Read the model definition and answer for the solid it produces. Units are mm, in the model's axes. Face numbers are marked on the shaded views. A direction names the side the tool comes from. Coordinates: 2 decimals unless noted, no trailing zeros. Order: outer loops, then holes, each group sorted by start corner. A loop starts at its lowest first (then second) coordinate and runs counter-clockwise, first axis right, second up. Notation, with made-up numbers: M -35.5,67.25 L -23.5,67.25 A20 cw -23.5,83.25 Z; hole C 89,-16.75 d9. An arc over 180 degrees is marked long. One line per question, with ' | ' between items. Start each with the question number.
1) A tool of negligible diameter and unlimited length cuts with its end or side. For the marked faces 1, 2 and 3, from which of +Z, -Z, +X, -X, +Y, -Y can it reach the whole face along a straight path? Write none if from no direction.
2) Find section D-D, the plane y = 0. Write down the section's boundary in (x, z), plus the area to 3 significant figures.
3) The mould has two halves that part along X. Classify the marked faces 4, 5 and 6: +X half, -X half, draft (parallel to the pull), parting line (faces both ways), or undercut.
4) Find section C-C, the plane x = 5. Write down the section's boundary in (y, z).
5) Given P1, Ø2, axis at x = 22, z = -2, coming from the -Y side; P2, Ø3, axis at x = 6, y = -0.5, coming from the -Z side; P3, Ø2, axis at y = 2, z = 5.5, coming from the -X side, each flat-ended and moving along its own axis, determine where each tip first touches the part or whether it passes through.
6) Consider probe 1 along X at (y, z) = (3.7, 0); probe 2 along X at (y, z) = (-4, -1.25); probe 3 along Z at (x, y) = (20, -2.95). Determine where each line is inside the solid, lowest interval first.
7) Find section B-B, the plane y = 2.5. Write down the section's boundary in (x, z), plus the area to 3 significant figures.
from build123d import *

# Parameters (mm, degrees)
SKETCH2_W           = 6
SKETCH2_H           = 10
BOSS_EXTRUDE1_DEPTH = 40
SKETCH3_R           = 11
BOSS_EXTRUDE2_DEPTH = 10
SKETCH4_R           = 7.5
CUT_EXTRUDE1_DEPTH  = 2
SKETCH6_R           = 3
CUT_EXTRUDE2_DEPTH  = 13
FILLET1_R           = 2
CUT_EXTRUDE3_REACH  = 44.673
SKETCH7_R           = 1.5


with BuildPart() as part:
    # Sketch2 → Boss-Extrude1 (new body)
    with BuildSketch(Plane(origin=(0, 0, 0), x_dir=(0, 0, -1), z_dir=(1, 0, 0))):
        Rectangle(SKETCH2_W, SKETCH2_H)
    extrude(amount=BOSS_EXTRUDE1_DEPTH)

    # Sketch3 → Boss-Extrude2 (add)
    with BuildSketch(Plane(origin=(0, 5, 0), x_dir=(1, 0, 0), z_dir=(0, 1, 0))):
        with Locations((20, 0)):
            Circle(SKETCH3_R)
    extrude(amount=-BOSS_EXTRUDE2_DEPTH)

    # Sketch4 → Cut-Extrude1 (cut)
    with BuildSketch(Plane(origin=(0, -5, 0), x_dir=(-1, 0, 0), z_dir=(0, -1, 0))):
        with Locations(Location((-20, 0, 0), (0, 0, 90))):
            Circle(SKETCH4_R)
    extrude(amount=-CUT_EXTRUDE1_DEPTH, mode=Mode.SUBTRACT)

    # Sketch5 → Cut-Revolve1 (revolve, cut)
    with BuildSketch(Plane(origin=(0, 0, 0), x_dir=(-1, 0, 0), z_dir=(0, 0, -1)), mode=Mode.PRIVATE) as cut_revolve1_sk:
        Polygon((-20, -3), (-27.5, -3), (-22.5, 2), (-20, 2), align=None)
    revolve(cut_revolve1_sk.sketch.rotate(Axis((20, 2, 0), (0, -1, 0)), 270), axis=Axis((20, 2, 0), (0, -1, 0)), mode=Mode.SUBTRACT)

    # Sketch6 → Cut-Extrude2 (cut)
    with BuildSketch(Plane.XZ.offset(-2)):
        with Locations(Location((20, 0, 0), (0, 0, 270))):
            Circle(SKETCH6_R)
    extrude(amount=-CUT_EXTRUDE2_DEPTH, mode=Mode.SUBTRACT)

    # Fillet1
    fillet1_edges = [part.edges().sort_by_distance(p)[0] for p in [
        (20, -5, 7.5),
    ]]
    fillet(fillet1_edges, radius=FILLET1_R - 0.0001)  # a hair under: the kernel refuses the full size

    # Sketch7 → Cut-Extrude3 (cut, up to next)
    with BuildSketch(Plane.XZ.offset(5), mode=Mode.PRIVATE) as cut_extrude3_sk1:
        with Locations(Location((5, 0, 0), (0, 0, 270))):
            Circle(SKETCH7_R)
    cut_extrude3_tool1 = extrude(cut_extrude3_sk1.sketch, amount=-CUT_EXTRUDE3_REACH, mode=Mode.PRIVATE) & part.part
    # Sketch7 → Cut-Extrude3 (cut, up to next)
    with BuildSketch(Plane.XZ.offset(5), mode=Mode.PRIVATE) as cut_extrude3_sk2:
        with Locations(Location((35, 0, 0), (0, 0, 270))):
            Circle(SKETCH7_R)
    cut_extrude3_tool2 = extrude(cut_extrude3_sk2.sketch, amount=-CUT_EXTRUDE3_REACH, mode=Mode.PRIVATE) & part.part
    add(cut_extrude3_tool1.solids().sort_by_distance((5, -5, 0))[0], mode=Mode.SUBTRACT)
    add(cut_extrude3_tool2.solids().sort_by_distance((35, -5, 0))[0], mode=Mode.SUBTRACT)


solid = part.part
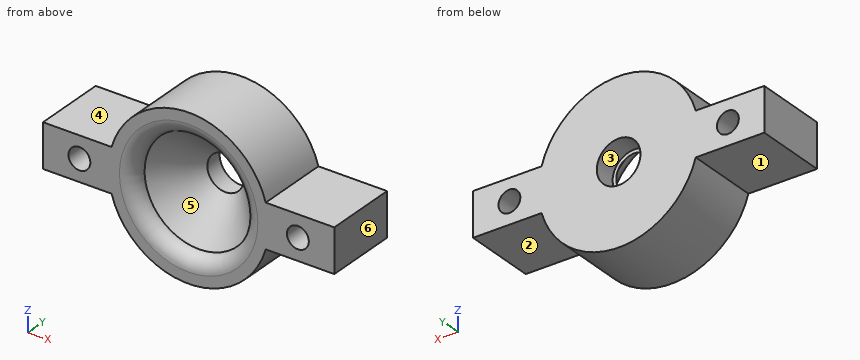
Report:
1) face 1: -Z, -X, +Y, -Y | face 2: -Z, +X, +Y, -Y | face 3: +Y
2) outline: M 0,-3 L 9.42,-3 A11 ccw 30.58,-3 L 40,-3 L 40,3 L 30.58,3 A11 ccw 9.42,3 L 0,3 Z; hole C 5,0 d3; hole C 20,0 d9; hole C 35,0 d3 | area: 412 mm^2
3) face 4: draft | face 5: undercut | face 6: +X half
4) outline: M -5,-3 L 5,-3 L 5,-1.5 L -5,-1.5 Z; M -5,1.5 L 5,1.5 L 5,3 L -5,3 Z
5) P1: stops at y = 0.67 | P2: stops at z = -3 | P3: stops at x = 9.96
6) probe 1: x = 0 to 3.5, 6.5 to 17, 23 to 33.5, 36.5 to 40 | probe 2: x = 0 to 4.17, 5.83 to 12.33, 27.67 to 34.17, 35.83 to 40 | probe 3: z = -11 to -7.45, 7.45 to 11
7) outline: M 0,-3 L 9.42,-3 A11 ccw 30.58,-3 L 40,-3 L 40,3 L 30.58,3 A11 ccw 9.42,3 L 0,3 Z; hole C 5,0 d3; hole C 20,0 d6; hole C 35,0 d3 | area: 447 mm^2
